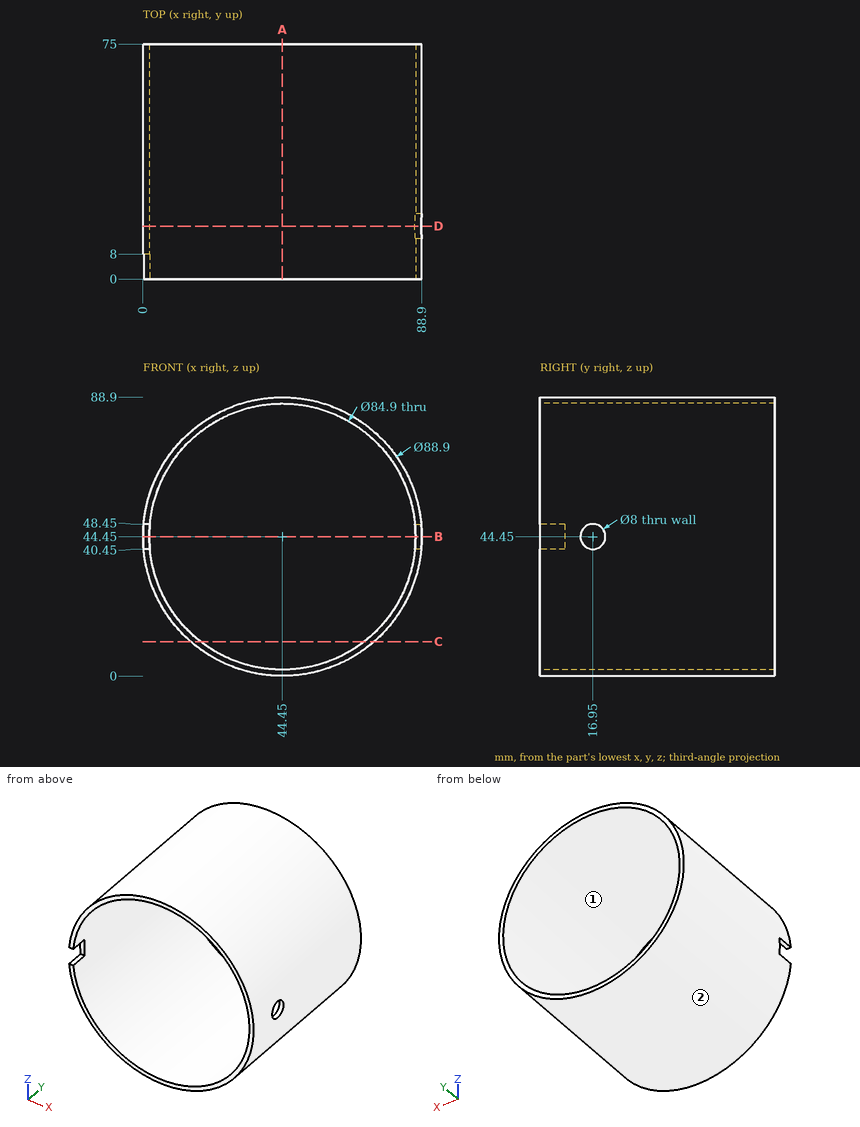
Answer from the drawing. Dimensions are ordinates in mm from the lowest x, y and z of the part. Give positions to 0.01 mm unless a question says otherwise; leave off trailing zeros. Loops run counter-clockwise (first coordinate to the right, second up) from the corner with the lowest first, then second, coordinate; pieces in that order, holes last. Notation, with made-up numbers: (19.5, 20.5) -> (26.5, 20.5) arc R22 ccw to (26.5, 58.5) -> close; hole circle Ø2 at (82, -22). An arc over 180 degrees is marked (long way). Use a Markdown table: item, result.
Q1. Section C-C, the plane z = 11 is taken. Determine the outline of the cut face in (x, y).
Solved:
| item | result |
|---|---|
| outline | (15.18, 0) -> (18.31, 0) -> (18.31, 75) -> (15.18, 75) -> close; (70.59, 0) -> (73.72, 0) -> (73.72, 75) -> (70.59, 75) -> close |
Q2. Section B-B, the plane z = 44.45 is taken. Determine the outline of the cut face in (x, y), then the cut area to 3 significant figures.
Solved:
| item | result |
|---|---|
| outline | (0, 8) -> (2, 8) -> (2, 75) -> (0, 75) -> close; (86.9, 0) -> (88.9, 0) -> (88.9, 12.95) -> (86.9, 12.95) -> close; (86.9, 20.95) -> (88.9, 20.95) -> (88.9, 75) -> (86.9, 75) -> close |
| area | 268 mm^2 |
Q3. Section A-A, the plane x = 44.45 is taken. Determine the outline of the cut face in (y, z).
Solved:
| item | result |
|---|---|
| outline | (0, 0) -> (75, 0) -> (75, 2) -> (0, 2) -> close; (0, 86.9) -> (75, 86.9) -> (75, 88.9) -> (0, 88.9) -> close |
Q4. Section D-D, the plane y = 16.95 is taken. Determine the outline of the cut face in (x, z), then the cut area to 3 significant figures.
Solved:
| item | result |
|---|---|
| outline | (86.71, 40.45) arc R42.45 cw (long way) to (86.71, 48.45) -> (88.72, 48.45) arc R44.45 ccw (long way) to (88.72, 40.45) -> close |
| area | 530 mm^2 |
Q5. Each of these flat-tipped pins is pushed along its axis until it touches: pin 1 (12 mm diameter, centred on y = 15, z = 22.5, fed in from +X); pin 2 (12 mm diameter, centred on y = 49.5, z = 41, fed in from +X); pin 3 (13 mm diameter, centred on y = 16.95, z = 44.45, fed in from -X). Where does it stop, or does it pass through?
Solved:
| item | result |
|---|---|
| pin 1 | stops at x = 85.94 |
| pin 2 | stops at x = 88.9 |
| pin 3 | stops at x = 0 |
Q6. Find the intervals of material crossed by line 1 along Y through (x, z) = (87, 44); line 2 along X through (y, z) = (22, 44.45), in increasing order.
Solved:
| item | result |
|---|---|
| line 1 | y = 0 to 12.98, 20.92 to 75 |
| line 2 | x = 0 to 2, 86.9 to 88.9 |
Q7. Determine the mould class of the marked faces 1 and 2 for opening direction Z: pulls with the +Z half, pulls with the -Z half, needs draft (parallel to the pull), parting line crosses it, or undercut.
Solved:
| item | result |
|---|---|
| face 1 | undercut |
| face 2 | parting line crosses it |
